Here's how the part is built. I have some questions about the finished solid (model axes, mm). Round coordinates to 2 decimals unless told otherwise and drop trailing zeros. Loops run counter-clockwise (first coordinate to the right, second up) from the corner with the lowest first, then second, coordinate; pieces in that order, holes last. Notation, with made-up numbers: M 3.5,42 L 13.5,42 A24 cw 13.5,64 Z; hole C -39,-40 d7. An arc over 180 degrees is marked long. Answer as a JSON object with one key per item and string values.
from build123d import *

# Parameters (mm, degrees)
BOSS_EXTRUDE1_DEPTH = 60
SKETCH3_R           = 45
CUT_EXTRUDE1_DEPTH  = 40
FILLET1_R           = 15


with BuildPart() as part:
    # Sketch2 → Boss-Extrude1 (new body)
    with BuildSketch(Plane(origin=(0, 0, 0), x_dir=(0, 0, -1), z_dir=(1, 0, 0))):
        Polygon((-60, 60), (-60, 120), (60, 120), (60, 60), (60, -60), (-60, -60), align=None)
    extrude(amount=BOSS_EXTRUDE1_DEPTH)

    # Sketch3 → Cut-Extrude1 (cut)
    with BuildSketch(Plane.ZY):
        Circle(SKETCH3_R)
    extrude(amount=-CUT_EXTRUDE1_DEPTH, mode=Mode.SUBTRACT)

    # Fillet1
    fillet1_edges = [part.edges().sort_by_distance(p)[0] for p in [
        (30, 120, 60),
        (30, 120, -60),
        (30, -60, -60),
        (30, -60, 60),
    ]]
    fillet(fillet1_edges, radius=FILLET1_R)


solid = part.part
Item 1: Please list where these lines run through material, in increasing order: probe 1 along Y at (x, z) = (13.5, 0); probe 2 along X at (y, z) = (17, -10); probe 3 along Y at (x, z) = (31, 32). Write a range as from..to.
Resolved:
{"probe 1": "-60..-45, 45..120", "probe 2": "40..60", "probe 3": "-60..-31.64, 31.64..120"}
Item 2: I want a section at A-A, the plane x = 27. Please give me the cut outline in (y, z).
Resolved:
{"outline": "M -60,-45 A15 ccw -45,-60 L 105,-60 A15 ccw 120,-45 L 120,45 A15 ccw 105,60 L -45,60 A15 ccw -60,45 Z; hole C 0,0 d90"}
Item 3: I want a section at C-C, the plane y = 0. Please give me the cut outline in (x, z), then the cut area to 3 significant figures.
Resolved:
{"outline": "M 0,-60 L 60,-60 L 60,60 L 0,60 L 0,45 L 40,45 L 40,-45 L 0,-45 Z", "area": "3,600 mm²"}
Item 4: I'm going to push a flat-ended pin straight in: pin 1 Ø2 at (y, z) = (3, 6.5) entering from -X. Where does the tip first touch, or does it pass through?
Resolved:
{"pin 1": "x = 40"}
Item 5: If we mould it in two halves opening along Z, with no side actions, what happens to faces 1 (the face through (30.42, 115.72, -55.49)), 2 (the face through (40, 1, -1)), 3 (the face through (30, 31, 60)), 4 (the face through (19.72, -39.923, 20.765))? For each: pulls with the +Z half, pulls with the -Z half, needs draft (parallel to the pull), parting line crosses it, or undercut.
Resolved:
{"face 1": "pulls with the -Z half", "face 2": "undercut", "face 3": "pulls with the +Z half", "face 4": "undercut"}
Item 6: I want a section at B-B, the plane z = 0. Please give me the cut outline in (x, y).
Resolved:
{"outline": "M 0,-60 L 60,-60 L 60,120 L 0,120 L 0,45 L 40,45 L 40,-45 L 0,-45 Z"}
